Here's how the part is built. I have some questions about the finished solid (model axes, mm). A direction names the side the tool comes from. Coordinates: 2 decimals unless noted, no trailing zeros. Write each loop counter-clockwise with the first axis right and the second up, starting at its lowest first coordinate (ties: lowest second). Pieces come first, ordered by that corner, then holes. Notation, with made-up numbers: (-8.5, 21.5) -> (42.5, 21.5) arc R19 ccw to (42.5, 38.5) -> close; hole circle Ø8 at (-16, 80.5). An arc over 180 degrees is marked (long way). Put each result on its own line as item: value. Start each with the question number.
Item 1: I need wall thicknesses on line 1 (Z direction, x = 7, y = 3.25); line 2 (X direction, y = -0.75, z = 2.75); line 3 (Y direction, x = 1.25, z = 1.75). Which ranges of each line are inside material? Lowest first, please. Write a range as [from, to].
Item 2: I want a section at A-A, the plane y = 0. List the corners of the cut face in (x, z) for me, then the cut area to 3 significant figures.
Item 3: I want a section at D-D, the plane z = 2. List the corners of the cut face in (x, y) for me.
Item 4: If we mould it in two halves opening along Y, with no side actions, what happens to faces 1 (the face through (7.99, -3.67, 4.78)), 2 (the face through (1.712, -1.978, -2.579)), 3 (the face through (-1, 2, -3)), 4 (the face through (4.5, 0, 0))? For each: released by +Y, released by -Y, zero draft, split by the parting line, or undercut.
Item 5: I want a section at C-C, the plane y = -4. List the corners of the cut face in (x, z) for me.
Item 6: On a 3-axis mill with a long thin cutter (end or side, diameter ignored), from which of +Z, -Z, +X, -X, +Y, -Y can I reach the whole of each face in a straight line? I mean faces 5 (the face through (8.5, 0, 0)), 6 (the face through (7.5, -3, -3)). Say none if no direction works.
Item 7: For pin 1 (4 mm diameter, centred on x = 1.5, z = -1, fed in from +Y); pin 2 (2 mm diameter, centred on y = -0.5, z = -0.5, fed in from -X); pin 3 (1.5 mm diameter, centred on x = 2.5, y = -2, fed in from -Z), each with a flat end and sliding along its axis, tell me the tip position at first contact or that it passes through.
from build123d import *

# Parameters (mm, degrees)
BASPROSKE_W             = 7.5
BASPROSKE_H             = 4.5
TOOTHCUT_DEPTH          = 10.836157786
TEETHCUTS_COUNT         = 16
TEETHCUTS_ANGLE         = 337.5
BORSKE_R                = 2.5
BORE_DEPTH              = 50.0000508
ESQUISSE5_R             = 6.027848577
ESQUISSE5_R_2           = 2.85
BOSS_EXTRU_4_DEPTH      = 1
BOSS_EXTRU_6_START      = -8.5
ESQUISSE7_R             = 3.00711341
BOSS_EXTRU_6_DEPTH      = 8.5
BOSS_EXTRU_7_START      = 1
BOSS_EXTRU_7_DEPTH      = 1
ESQUISSE9_R             = 3.25
ENL_V_MAT_EXTRU_1_DEPTH = 5.5


with BuildPart() as part:
    # BasProSke → Base-Revolve (revolve)
    with BuildSketch(Plane(origin=(0, 0, 0), x_dir=(1, 0, 0), z_dir=(0, 1, 0)), mode=Mode.PRIVATE) as base_revolve_sk:
        with Locations((3.75, 2.25)):
            Rectangle(BASPROSKE_W, BASPROSKE_H)
    revolve(base_revolve_sk.sketch.rotate(Axis((-10, 0, 0), (1, 0, 0)), 180), axis=Axis((-10, 0, 0), (1, 0, 0)))

    # TooCutSke → ToothCut (cut, through all)
    with BuildSketch(Plane(origin=(0, 0, 0), x_dir=(0, 0, -1), z_dir=(1, 0, 0))):
        with BuildLine():
            ThreePointArc((0.306025637, 3.360092902), (0, 3.374), (-0.306025637, 3.360092902))
            ThreePointArc((-0.306025637, 3.360092902), (-0.415941512, 3.953968919), (-0.738171669, 4.464789776))
            ThreePointArc((-0.738171669, 4.464789776), (0, 4.5254), (0.738171669, 4.464789776))
            ThreePointArc((0.738171669, 4.464789776), (0.415941512, 3.953968919), (0.306025637, 3.360092902))
        make_face()
    toothcut = extrude(amount=TOOTHCUT_DEPTH, mode=Mode.SUBTRACT)

    # TeethCuts: ToothCut ×16 about axis
    teethcuts_axis = Axis((-10, 0, 0), (1, 0, 0))
    for i in range(1, TEETHCUTS_COUNT):
        add(toothcut.rotate(teethcuts_axis, i * TEETHCUTS_ANGLE / (TEETHCUTS_COUNT - 1)), mode=Mode.SUBTRACT)

    # BorSke → Bore (cut, symmetric)
    with BuildSketch(Plane(origin=(0, 0, 0), x_dir=(0, 0, -1), z_dir=(1, 0, 0))):
        with Locations(Location((0, 0, 0), (0, 0, 180))):
            Circle(BORSKE_R)
    extrude(amount=BORE_DEPTH, both=True, mode=Mode.SUBTRACT)

    # Esquisse5 → Boss.-Extru.4 (add)
    with BuildSketch(Plane(origin=(7.5, 0, 0), x_dir=(0, 0, -1), z_dir=(1, 0, 0))):
        Circle(ESQUISSE5_R)
        Circle(ESQUISSE5_R_2, mode=Mode.SUBTRACT)
    extrude(amount=BOSS_EXTRU_4_DEPTH)

    # Esquisse7 → Boss.-Extru.6 (add)
    with BuildSketch(Plane.ZY.offset(BOSS_EXTRU_6_START)):
        Circle(ESQUISSE7_R)
    extrude(amount=BOSS_EXTRU_6_DEPTH)

    # Esquisse8 → Boss.-Extru.7 (add)
    with BuildSketch(Plane.ZY.offset(BOSS_EXTRU_7_START)):
        with BuildLine():
            ThreePointArc((3.360092902, 0.306025637), (3.939792443, 0.410473293), (4.442413227, 0.717610424))
            ThreePointArc((4.442413227, 0.717610424), (4.413533762, 0.877906449), (4.378872276, 1.037052359))
            ThreePointArc((4.378872276, 1.037052359), (3.796974929, 1.128465421), (3.221432001, 1.003121062))
            ThreePointArc((3.221432001, 1.003121062), (3.117169543, 1.291173901), (2.987210118, 1.568582707))
            ThreePointArc((2.987210118, 1.568582707), (3.482812272, 1.886921168), (3.829637035, 2.363023525))
            ThreePointArc((3.829637035, 2.363023525), (3.741613255, 2.500066049), (3.648687715, 2.633833321))
            ThreePointArc((3.648687715, 2.633833321), (3.076102401, 2.495605504), (2.59233728, 2.159551673))
            ThreePointArc((2.59233728, 2.159551673), (2.38577828, 2.38577828), (2.159551673, 2.59233728))
            ThreePointArc((2.159551673, 2.59233728), (2.495605504, 3.076102401), (2.633833321, 3.648687715))
            ThreePointArc((2.633833321, 3.648687715), (2.500066049, 3.741613255), (2.363023525, 3.829637035))
            ThreePointArc((2.363023525, 3.829637035), (1.886921168, 3.482812272), (1.568582707, 2.987210118))
            ThreePointArc((1.568582707, 2.987210118), (1.291173901, 3.117169543), (1.003121062, 3.221432001))
            ThreePointArc((1.003121062, 3.221432001), (1.128465421, 3.796974929), (1.037052359, 4.378872276))
            ThreePointArc((1.037052359, 4.378872276), (0.877906449, 4.413533762), (0.717610424, 4.442413227))
            ThreePointArc((0.717610424, 4.442413227), (0.410473293, 3.939792443), (0.306025637, 3.360092902))
            ThreePointArc((0.306025637, 3.360092902), (0, 3.374), (-0.306025637, 3.360092902))
            ThreePointArc((-0.306025637, 3.360092902), (-0.410473293, 3.939792443), (-0.717610424, 4.442413227))
            ThreePointArc((-0.717610424, 4.442413227), (-0.877906449, 4.413533762), (-1.037052359, 4.378872276))
            ThreePointArc((-1.037052359, 4.378872276), (-1.128465421, 3.796974929), (-1.003121062, 3.221432001))
            ThreePointArc((-1.003121062, 3.221432001), (-1.291173901, 3.117169543), (-1.568582707, 2.987210118))
            ThreePointArc((-1.568582707, 2.987210118), (-1.886921168, 3.482812272), (-2.363023525, 3.829637035))
            ThreePointArc((-2.363023525, 3.829637035), (-2.500066049, 3.741613255), (-2.633833321, 3.648687715))
            ThreePointArc((-2.633833321, 3.648687715), (-2.495605504, 3.076102401), (-2.159551673, 2.59233728))
            ThreePointArc((-2.159551673, 2.59233728), (-2.38577828, 2.38577828), (-2.59233728, 2.159551673))
            ThreePointArc((-2.59233728, 2.159551673), (-3.076102401, 2.495605504), (-3.648687715, 2.633833321))
            ThreePointArc((-3.648687715, 2.633833321), (-3.741613255, 2.500066049), (-3.829637035, 2.363023525))
            ThreePointArc((-3.829637035, 2.363023525), (-3.482812272, 1.886921168), (-2.987210118, 1.568582707))
            ThreePointArc((-2.987210118, 1.568582707), (-3.117169543, 1.291173901), (-3.221432001, 1.003121062))
            ThreePointArc((-3.221432001, 1.003121062), (-3.796974929, 1.128465421), (-4.378872276, 1.037052359))
            ThreePointArc((-4.378872276, 1.037052359), (-4.413533762, 0.877906449), (-4.442413227, 0.717610424))
            ThreePointArc((-4.442413227, 0.717610424), (-3.939792443, 0.410473293), (-3.360092902, 0.306025637))
            ThreePointArc((-3.360092902, 0.306025637), (-3.374, 0), (-3.360092902, -0.306025637))
            ThreePointArc((-3.360092902, -0.306025637), (-3.939792443, -0.410473293), (-4.442413227, -0.717610424))
            ThreePointArc((-4.442413227, -0.717610424), (-4.413533762, -0.877906449), (-4.378872276, -1.037052359))
            ThreePointArc((-4.378872276, -1.037052359), (-3.796974929, -1.128465421), (-3.221432001, -1.003121062))
            ThreePointArc((-3.221432001, -1.003121062), (-3.117169543, -1.291173901), (-2.987210118, -1.568582707))
            ThreePointArc((-2.987210118, -1.568582707), (-3.482812272, -1.886921168), (-3.829637035, -2.363023525))
            ThreePointArc((-3.829637035, -2.363023525), (-3.741613255, -2.500066049), (-3.648687715, -2.633833321))
            ThreePointArc((-3.648687715, -2.633833321), (-3.076102401, -2.495605504), (-2.59233728, -2.159551673))
            ThreePointArc((-2.59233728, -2.159551673), (-2.38577828, -2.38577828), (-2.159551673, -2.59233728))
            ThreePointArc((-2.159551673, -2.59233728), (-2.495605504, -3.076102401), (-2.633833321, -3.648687715))
            ThreePointArc((-2.633833321, -3.648687715), (-2.500066049, -3.741613255), (-2.363023525, -3.829637035))
            ThreePointArc((-2.363023525, -3.829637035), (-1.886921168, -3.482812272), (-1.568582707, -2.987210118))
            ThreePointArc((-1.568582707, -2.987210118), (-1.291173901, -3.117169543), (-1.003121062, -3.221432001))
            ThreePointArc((-1.003121062, -3.221432001), (-1.128465421, -3.796974929), (-1.037052359, -4.378872276))
            ThreePointArc((-1.037052359, -4.378872276), (-0.877906449, -4.413533762), (-0.717610424, -4.442413227))
            ThreePointArc((-0.717610424, -4.442413227), (-0.410473293, -3.939792443), (-0.306025637, -3.360092902))
            ThreePointArc((-0.306025637, -3.360092902), (0, -3.374), (0.306025637, -3.360092902))
            ThreePointArc((0.306025637, -3.360092902), (0.410473293, -3.939792443), (0.717610424, -4.442413227))
            ThreePointArc((0.717610424, -4.442413227), (0.877906449, -4.413533762), (1.037052359, -4.378872276))
            ThreePointArc((1.037052359, -4.378872276), (1.128465421, -3.796974929), (1.003121062, -3.221432001))
            ThreePointArc((1.003121062, -3.221432001), (1.291173901, -3.117169543), (1.568582707, -2.987210118))
            ThreePointArc((1.568582707, -2.987210118), (1.886921168, -3.482812272), (2.363023525, -3.829637035))
            ThreePointArc((2.363023525, -3.829637035), (2.500066049, -3.741613255), (2.633833321, -3.648687715))
            ThreePointArc((2.633833321, -3.648687715), (2.495605504, -3.076102401), (2.159551673, -2.59233728))
            ThreePointArc((2.159551673, -2.59233728), (2.38577828, -2.38577828), (2.59233728, -2.159551673))
            ThreePointArc((2.59233728, -2.159551673), (3.076102401, -2.495605504), (3.648687715, -2.633833321))
            ThreePointArc((3.648687715, -2.633833321), (3.741613255, -2.500066049), (3.829637035, -2.363023525))
            ThreePointArc((3.829637035, -2.363023525), (3.482812272, -1.886921168), (2.987210118, -1.568582707))
            ThreePointArc((2.987210118, -1.568582707), (3.117169543, -1.291173901), (3.221432001, -1.003121062))
            ThreePointArc((3.221432001, -1.003121062), (3.796974929, -1.128465421), (4.378872276, -1.037052359))
            ThreePointArc((4.378872276, -1.037052359), (4.413533762, -0.877906449), (4.442413227, -0.717610424))
            ThreePointArc((4.442413227, -0.717610424), (3.939792443, -0.410473293), (3.360092902, -0.306025637))
            ThreePointArc((3.360092902, -0.306025637), (3.374, 0), (3.360092902, 0.306025637))
        make_face()
    extrude(amount=-BOSS_EXTRU_7_DEPTH)

    # Esquisse9 → Enlèv. mat.-Extru.1 (cut)
    with BuildSketch(Plane.ZY.offset(1)):
        Circle(ESQUISSE9_R)
    extrude(amount=-ENL_V_MAT_EXTRU_1_DEPTH, mode=Mode.SUBTRACT)


solid = part.part
Calculated:
1. line 1: z = [-2.56, -1.7], [-1.01, 1.01], [1.7, 2.56]
1. line 2: x = [4.5, 8.5]
1. line 3: y = [-3.32, -2.74], [2.74, 3.32]
2. outline: (-1, -3.37) -> (7.5, -3.37) -> (7.5, -6.03) -> (8.5, -6.03) -> (8.5, 6.03) -> (7.5, 6.03) -> (7.5, 3.37) -> (-1, 3.37) -> (-1, 3.25) -> (4.5, 3.25) -> (4.5, -3.25) -> (-1, -3.25) -> close
2. area: 33.7 mm2
3. outline: (-1, -3.59) -> (7.5, -3.59) -> (7.5, -5.69) -> (8.5, -5.69) -> (8.5, 5.69) -> (7.5, 5.69) -> (7.5, 3.59) -> (-1, 3.59) -> (-1, 2.56) -> (4.5, 2.56) -> (4.5, -2.56) -> (-1, -2.56) -> close
4. face 1: split by the parting line
4. face 2: undercut
4. face 3: zero draft
4. face 4: undercut
5. outline: (-1, -1.12) -> (7.5, -1.12) -> (7.5, -4.51) -> (8.5, -4.51) -> (8.5, 4.51) -> (7.5, 4.51) -> (7.5, 1.12) -> (-1, 1.12) -> (-1, 0.43) -> (7.5, 0.43) -> (7.5, -0.43) -> (-1, -0.43) -> close
6. face 5: +Z, -Z, +X, +Y, -Y
6. face 6: -X
7. pin 1: stops at y = 4.44
7. pin 2: stops at x = 4.5
7. pin 3: stops at z = -3.83
